Source: CAD feature listing. Evaluate the final solid. Frame: model axes, mm. Give positions to 0.01 mm unless a question says otherwise; leave off trailing zeros. Order: outer loops, then holes, each group sorted by start corner. A loop starts at its lowest first (then second) coordinate and runs counter-clockwise, first axis right, second up.
1) Draft query along X for faces 1 (the face through (232.11, -9, 3)), 2 (the face through (78, -7, 6.35)), 3 (the face through (67.938, -3.88, 3.219)). Return one class per face: released by +X, released by -X, zero draft, split by the parting line, or undercut.
2) Material intervals for line 1 (Y direction, x = 193, z = 5.75); line 2 (X direction, y = -7, z = 4.75); line 3 (X direction, y = -1, z = 0.5), sorted ascending.
3) Section A-A, the plane y = -15.5. Return loops of the section in (x, z), plus the area to 3 significant figures.
4) Section B-B, the plane z = 2.25. Give the number of separate pieces and of enclosed holes in the cut face, plus the area to 3 significant figures.
```python
from build123d import *

# Parameters (mm, degrees)
F0_W      = 304.8
F0_H      = 101.6
F1_DEPTH  = 6.35
F2_R      = 3.175
F3_DEPTH  = 6.35
F4_R      = 14.2875
F5_DEPTH  = 6.35
F6_R      = 14.2875
F7_DEPTH  = 6.35
F9_R      = 2.413
F10_DEPTH = 6.35
F11_R     = 3.0861
F12_DEPTH = 6.35
F13_R     = 3.0861
F14_DEPTH = 6.35
F15_R     = 3.0861
F16_DEPTH = 6.35


with BuildPart() as f1:
    # F0 (on Top) → F1 (new body)
    with BuildSketch(Plane.XY):
        with Locations((79.710026, -8.171286)):
            Rectangle(F0_W, F0_H)
    extrude(amount=F1_DEPTH)

    # F2 (on face) → F3 (cut)
    with BuildSketch(Plane.XY.offset(6.35)):
        with Locations((-47.289974, -8.171286)):
            Circle(F2_R)
    extrude(amount=-F3_DEPTH, mode=Mode.SUBTRACT)

    # F4 (on face) → F5 (cut)
    with BuildSketch(Plane.XY.offset(6.35)):
        with Locations((194.010026, -8.171286)):
            Circle(F4_R)
    extrude(amount=-F5_DEPTH, mode=Mode.SUBTRACT)

    # F6 (on face) → F7 (cut)
    with BuildSketch(Plane.XY.offset(6.35)):
        with Locations((54.310026, -8.171286)):
            Circle(F6_R)
    extrude(amount=-F7_DEPTH, mode=Mode.SUBTRACT)

    # F9 (on face) → F10 (cut)
    with BuildSketch(Plane.XY.offset(6.35)):
        with Locations((36.580826, -25.900486)):
            Circle(F9_R)
        with Locations((72.039226, 9.557914)):
            Circle(F9_R)
    extrude(amount=-F10_DEPTH, mode=Mode.SUBTRACT)

    # F11 (on face) → F12 (cut)
    with BuildSketch(Plane.XY):
        with Locations((105.110026, -8.171286)):
            Circle(F11_R)
    extrude(amount=F12_DEPTH, mode=Mode.SUBTRACT)

    # F13 (on face) → F14 (cut)
    with BuildSketch(Plane.XY):
        with Locations((27.322526, 29.928714)):
            Circle(F13_R)
    extrude(amount=F14_DEPTH, mode=Mode.SUBTRACT)

    # F15 (on face) → F16 (cut)
    with BuildSketch(Plane.XY.offset(6.35)):
        with Locations((219.410026, 29.928714)):
            Circle(F15_R)
    extrude(amount=-F16_DEPTH, mode=Mode.SUBTRACT)


solid = f1.part
```
From the geometry:
1. face 1: released by +X
1. face 2: zero draft
1. face 3: undercut
2. line 1: y = -58.97 to -22.42, 6.08 to 42.63
2. line 2: x = -72.69 to -50.24, -44.34 to 40.07, 68.55 to 102.25, 107.97 to 179.77, 208.25 to 232.11
2. line 3: x = -72.69 to 41.95, 66.67 to 181.65, 206.37 to 232.11
3. outline: (-72.69, 0) - (42.05, 0) - (42.05, 6.35) - (-72.69, 6.35) - close; (66.57, 0) - (181.75, 0) - (181.75, 6.35) - (66.57, 6.35) - close; (206.27, 0) - (232.11, 0) - (232.11, 6.35) - (206.27, 6.35) - close
3. area: 1,620 mm2
4. separate pieces: 1
4. enclosed holes: 8
4. area: 29,500 mm2
